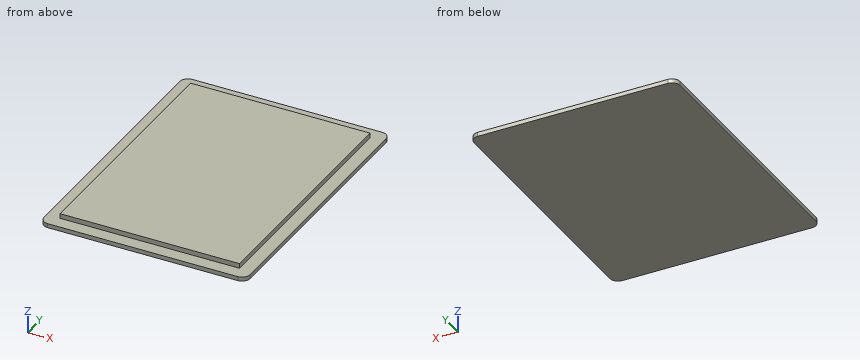
from build123d import *

# Parameters (mm, degrees)
SKETCH_1_W      = 471
SKETCH_1_H      = 626
EXTRUDE_1_DEPTH = 4.75
FILLET_1_R      = 18
SKETCH_2_W      = 411
SKETCH_2_H      = 566
EXTRUDE_2_DEPTH = 11


with BuildPart() as part:
    # Эскиз1 → Бобышка-Вытянуть1 (new, symmetric)
    with BuildSketch(Plane.XY):
        Rectangle(SKETCH_1_W, SKETCH_1_H)
    extrude(amount=EXTRUDE_1_DEPTH, both=True)

    # Скругление1
    fillet_1_edges = [part.edges().sort_by_distance(p)[0] for p in [
        (235.5, -313, 0),
        (-235.5, -313, 0),
        (-235.5, 313, 0),
        (235.5, 313, 0),
    ]]
    fillet(fillet_1_edges, radius=FILLET_1_R)

    # Эскиз2 → Бобышка-Вытянуть2 (add)
    with BuildSketch(Plane.XY.offset(4.75)):
        Rectangle(SKETCH_2_W, SKETCH_2_H)
    extrude(amount=EXTRUDE_2_DEPTH)


solid = part.part
For this review, take the finished solid that the model builds, in its own axes (mm). Round coordinates to 2 decimals unless told otherwise and drop trailing zeros. Order: outer loops, then holes, each group sorted by start corner. A loop starts at its lowest first (then second) coordinate and runs counter-clockwise, first axis right, second up. Notation, with made-up numbers: M 64,-17.5 L 87,-17.5 A17 ccw 87,-12.5 Z; hole C 77,17 d8. An arc over 180 degrees is marked long. Write each question's results on one line, items separated by ' | '. Start each with the question number.
1. Add section C-C (z = 11.5). State the section outline as (x, y) points, then the cut area to 3 significant figures.
2. Add section B-B (x = -18). State the section outline as (y, z) points.
3. Add section A-A (y = -73). State the section outline as (x, z) points.
4. Clearance check with flat-ended pins moving along their axes: pin 1 Ø12 at (y, z) = (-134, 10.5) entering from -X; pin 2 Ø12 at (y, z) = (212.5, 12) entering from -X; pin 3 Ø3.5 at (x, z) = (17.5, 11) entering from -Y; pin 4 Ø2 at (x, z) = (-103.5, 11.5) entering from +Y. State where each tip first meets the part, or that it passes through.
5. To check wall thickness, follow L1, parallel to Y at x = 24, z = 6.5; L2, parallel to X at y = -6.5, z = 7.75. State the ranges of each line that lie inside material, in increasing order. Write a range as [from, to].
Output values:
1) outline: M -205.5,-283 L 205.5,-283 L 205.5,283 L -205.5,283 Z | area: 233,000 mm^2
2) outline: M -313,-4.75 L 313,-4.75 L 313,4.75 L 283,4.75 L 283,15.75 L -283,15.75 L -283,4.75 L -313,4.75 Z
3) outline: M -235.5,-4.75 L 235.5,-4.75 L 235.5,4.75 L 205.5,4.75 L 205.5,15.75 L -205.5,15.75 L -205.5,4.75 L -235.5,4.75 Z
4) pin 1: x = -235.5 | pin 2: x = -205.5 | pin 3: y = -283 | pin 4: y = 283
5) L1: [-283, 283] | L2: [-205.5, 205.5]
